```python
from build123d import *

# Parameters (mm, degrees)
F1_DEPTH = 6
F2_SIZE  = 1.99999


# Not quite as in the source:
# - a fillet or chamfer is up to 0.001 mm smaller than in the source, because OpenCascade refuses the exact size


with BuildPart() as f1:
    # F0 (on Top) → F1 (new body)
    with BuildSketch(Plane.XY):
        Polygon((-4, 7), (-4, 2), (-30, 2), (-30, 6), (-32, 6), (-32, 0), (0, 0), (0, 7), align=None)
    extrude(amount=F1_DEPTH)

    # F2 (size 2 in the source; OpenCascade refuses exactly that, so slightly less here)
    f2_edges = [f1.edges().sort_by_distance(p)[0] for p in [
        (-32, 6, 3),
    ]]
    chamfer(f2_edges, length=F2_SIZE)


solid = f1.part
```
The listing builds one solid part. Answer for the finished solid, in the listing's coordinates (mm). A direction names the side the tool comes from. Coordinates: 2 decimals unless noted, no trailing zeros. Order: outer loops, then holes, each group sorted by start corner. A loop starts at its lowest first (then second) coordinate and runs counter-clockwise, first axis right, second up. Notation, with made-up numbers: M 15,50.5 L 34,50.5 A18 cw 34,72.5 Z; hole C 83,83.5 d11. An arc over 180 degrees is marked long. Answer as a JSON object with one key per item and string values. Group by question number.
1. Determine the mould class of faces 1 (the flat face through (-4, 5, 3)), 2 (the flat face through (-2, 7, 3)), 3 (the flat face through (-31, 5, 3)) for opening direction X: released by +X, released by -X, zero draft, split by the parting line, or undercut.
2. Section C-C on x = -20 is taken. Write down the section's boundary in (y, z), then the cut area to 3 significant figures.
3. A flat-ended cylindrical pin translates along its axis: P1, Ø1.8, axis at x = -20.5, z = 4, coming from the +Y side. Find the tip coordinate at first contact, or state that the pin passes through.
4. Section A-A on y = 2.5 is taken. Write down the section's boundary in (x, z), then the cut area to 3 significant figures.
5. A tool of negligible diameter and unlimited length cuts with its end or side. For faces 4 (the flat face through (-16, 1, 0)), 5 (the flat face through (-17, 2, 3)), from which of +Z, -Z, +X, -X, +Y, -Y can it reach the whole face along a straight path? Write none if from no direction.
6. Straight lines are drawn through the part: line 1 (X direction, y = 3, z = 0.75); line 2 (Y direction, x = -14, z = 5); line 3 (X direction, y = 5.25, z = 1). For each, find the intervals that lie inside material, in ascending order.
Values follow:
{
 "1": {"face 1": "undercut", "face 2": "zero draft", "face 3": "released by -X"},
 "2": {"outline": "M 0,0 L 2,0 L 2,6 L 0,6 Z", "area": "12.0 mm2"},
 "3": {"P1": "y = 2"},
 "4": {"outline": "M -32,0 L -30,0 L -30,6 L -32,6 Z; M -4,0 L 0,0 L 0,6 L -4,6 Z", "area": "36.0 mm2"},
 "5": {"face 4": "-Z, +X, -X, +Y, -Y", "face 5": "+Z, -Z, +Y"},
 "6": {"line 1": "-32 to -30, -4 to 0", "line 2": "0 to 2", "line 3": "-30.75 to -30, -4 to 0"}
}
